```python
from build123d import *

# Parameters (mm, degrees)
SKETCH_1_W                   = 60
SKETCH_1_H                   = 20
EXTRUDE_1_DEPTH              = 20
SKETCH_2_W                   = 60
SKETCH_2_H                   = 40
EXTRUDE_2_DEPTH              = 5
SKETCH_3_W                   = 20
SKETCH_3_H                   = 5
EXTRUDE_3_DEPTH              = 20
HOLE_WIZARD_M4_2_D           = 4.5
HOLE_WIZARD_M4_2_CBORE_D     = 8
HOLE_WIZARD_M4_2_CBORE_DEPTH = 4
SKETCH_8_W                   = 15
SKETCH_8_H                   = 20
CUT_EXTRUDE_1_DEPTH          = 84.815273071
HOLE_WIZARD_M4_1_D           = 4.5
HOLE_WIZARD_M4_1_CBORE_D     = 8
HOLE_WIZARD_M4_1_CBORE_DEPTH = 4
SKETCH_10_W                  = 60
SKETCH_10_H                  = 5
EXTRUDE_4_DEPTH              = 80
SKETCH_11_W                  = 60
SKETCH_11_H                  = 5
EXTRUDE_5_DEPTH              = 20
FILLET_1_R                   = 20
SKETCH_12_W                  = 10
SKETCH_12_H                  = 5
CUT_EXTRUDE_2_DEPTH          = 129.937969582
SKETCH_13_W                  = 14
SKETCH_13_H                  = 20
CUT_EXTRUDE_3_DEPTH          = 35
SKETCH_14_W                  = 14
SKETCH_14_H                  = 3
EXTRUDE_6_DEPTH              = 20
HOLE_WIZARD_M4_1_2_D         = 4.6
HOLE_WIZARD_M4_1_2_DEPTH     = 5


with BuildPart() as part:
    # 스케치1 → 보스-돌출1 (new body)
    with BuildSketch(Plane.XY):
        Rectangle(SKETCH_1_W, SKETCH_1_H)
    extrude(amount=EXTRUDE_1_DEPTH)

    # 스케치2 → 보스-돌출2 (add)
    with BuildSketch(Plane.XZ.offset(10)):
        Rectangle(SKETCH_2_W, SKETCH_2_H)
    extrude(amount=EXTRUDE_2_DEPTH)

    # 스케치3 → 보스-돌출3 (add)
    with BuildSketch(Plane(origin=(30, 0, 0), x_dir=(0, 0, -1), z_dir=(1, 0, 0))):
        with Locations((10, -12.5)):
            Rectangle(SKETCH_3_W, SKETCH_3_H)
    extrude_3 = extrude(amount=EXTRUDE_3_DEPTH)

    # 대칭 복사1: 보스-돌출3 across plane
    add(extrude_3.mirror(Plane.ZY))

    # M4 소켓 머리 캡 나사용 카운터보어2 (through all)
    with Locations(Plane(origin=(0, -15, 0), x_dir=(-1, 0, 0), z_dir=(0, -1, 0))):
        with Locations((40, 10), (-40, 10)):
            CounterBoreHole(HOLE_WIZARD_M4_2_D / 2, HOLE_WIZARD_M4_2_CBORE_D / 2, HOLE_WIZARD_M4_2_CBORE_DEPTH)

    # 스케치8 → 컷-돌출1 (cut, through all)
    with BuildSketch(Plane(origin=(30, 0, 0), x_dir=(0, 0, -1), z_dir=(1, 0, 0))):
        with Locations((-12.5, 0)):
            Rectangle(SKETCH_8_W, SKETCH_8_H)
    extrude(amount=-CUT_EXTRUDE_1_DEPTH, mode=Mode.SUBTRACT)

    # Hole Wizard M4 _ _ _ _ _1 (through all)
    with Locations(Plane(origin=(0, -10, 0), x_dir=(1, 0, 0), z_dir=(0, 1, 0))):
        with Locations((-15, 10), (15, 10), (-15, -10), (15, -10)):
            CounterBoreHole(HOLE_WIZARD_M4_1_D / 2, HOLE_WIZARD_M4_1_CBORE_D / 2, HOLE_WIZARD_M4_1_CBORE_DEPTH)

    # 스케치10 → 보스-돌출4 (add)
    with BuildSketch(Plane.XY.offset(20)):
        with Locations((0, -12.5)):
            Rectangle(SKETCH_10_W, SKETCH_10_H)
    extrude(amount=EXTRUDE_4_DEPTH)

    # 스케치11 → 보스-돌출5 (add)
    with BuildSketch(Plane(origin=(0, -10, 0), x_dir=(1, 0, 0), z_dir=(0, 1, 0))):
        with Locations((0, -97.5)):
            Rectangle(SKETCH_11_W, SKETCH_11_H)
    extrude(amount=EXTRUDE_5_DEPTH)

    # 필렛1
    fillet_1_edges = [part.edges().sort_by_distance(p)[0] for p in [
        (0, -10, 95),
    ]]
    fillet(fillet_1_edges, radius=FILLET_1_R - 0.0001)  # a hair under: the kernel refuses the full size

    # 스케치12 → 컷-돌출2 (cut, through all)
    with BuildSketch(Plane.ZY.offset(30)):
        with Locations((95, -12.5)):
            Rectangle(SKETCH_12_W, SKETCH_12_H)
    extrude(amount=-CUT_EXTRUDE_2_DEPTH, mode=Mode.SUBTRACT)

    # 스케치13 → 컷-돌출3 (cut)
    with BuildSketch(Plane.XY.offset(60)):
        with Locations((-15, 0)):
            Rectangle(SKETCH_13_W, SKETCH_13_H)
        with Locations((15, 0)):
            Rectangle(SKETCH_13_W, SKETCH_13_H)
    extrude(amount=CUT_EXTRUDE_3_DEPTH, mode=Mode.SUBTRACT)

    # 스케치14 → 보스-돌출6 (add)
    with BuildSketch(Plane(origin=(0, 0, 95), x_dir=(-1, 0, 0), z_dir=(0, 0, -1))):
        with Locations((-15, -8.5)):
            Rectangle(SKETCH_14_W, SKETCH_14_H)
        with Locations((15, -8.5)):
            Rectangle(SKETCH_14_W, SKETCH_14_H)
    extrude(amount=EXTRUDE_6_DEPTH)

    # Hole Wizard M4 _ _1 2
    with Locations(Plane(origin=(0, 0, 95), x_dir=(-1, 0, 0), z_dir=(0, 0, -1))):
        with Locations((-15, 0), (15, 0)):
            Hole(HOLE_WIZARD_M4_1_2_D / 2, depth=HOLE_WIZARD_M4_1_2_DEPTH)


solid = part.part
```
Part model, mm, in its own coordinate system. A direction names the side the tool comes from. Round coordinates to 2 decimals unless told otherwise and drop trailing zeros. Loops run counter-clockwise (first coordinate to the right, second up) from the corner with the lowest first, then second, coordinate; pieces in that order, holes last. Notation, with made-up numbers: (30, 8.25) -> (47, 8.25) arc R13 ccw to (47, 20.25) -> close; hole circle Ø5 at (-16.75, 56). An arc over 180 degrees is marked (long way). Use one line per item in the form item = value. Start each with the question number.
Item 1: Band-saw the part on A-A (z = 10). List the corners of the cut face in (x, y), plus the area to 3 significant figures.
Item 2: Band-saw the part on B-B (x = -15). Give the number of separate pieces and of enclosed holes in the cut face, plus the area to 3 significant figures.
Item 3: Band-saw the part on D-D (y = -5.5). List the corners of the cut face in (x, z).
Item 4: Tool access for faces 4 (the flat face through (0, 0, 0)), 5 (the flat face through (-22, -8, 79)), 6 (the cylindrical face through (-36, -13, -10)): list every direction of +Z, -Z, +X, -X, +Y, -Y with a clear straight run to the whole face (end or side of a thin tool).
Item 5: Two-plate mould, pull along X, no slides. Class faces 1 (the flat face through (22, -8, 79)), 2 (the cylindrical face through (11, -12, -10)), 3 (the flat face through (0, -10, 40)): released by +X, released by -X, zero draft, split by the parting line, or undercut.
Item 6: Drill centre lines: line 1 along Z through (x, y) = (15, -12.85); line 2 along X through (y, z) = (-14.45, 10); line 3 along Y through (x, z) = (15, 97.05). Where is each one in solid material? Low to high.
Item 7: Drop flat-ended pins along their axis: pin 1 Ø4 at (x, y) = (-45, -12) entering from +Z; pin 2 Ø5 at (x, y) = (-0.5, 2.5) entering from -Z; pin 3 Ø8 at (x, z) = (3.5, 39) entering from +Y; pin 4 Ø10.5 at (x, z) = (-40, -10) entering from -Y. Give the stop position or say it passes through.
Item 8: Band-saw the part on C-C (x = 40). List the corners of the cut face in (y, z), plus the area to 3 significant figures.
Data:
q1.outline = (-30, -15) -> (-17.25, -15) -> (-17.25, -14) -> (-19, -14) -> (-19, -10) -> (-30, -10) -> close; (-12.75, -15) -> (12.75, -15) -> (12.75, -14) -> (11, -14) -> (11, -10) -> (-11, -10) -> (-11, -14) -> (-12.75, -14) -> close; (17.25, -15) -> (30, -15) -> (30, -10) -> (19, -10) -> (19, -14) -> (17.25, -14) -> close
q1.area = 227 mm^2
q2.separate_pieces = 4
q2.enclosed_holes = 0
q2.area = 714 mm^2
q3.outline = (-30, 0) -> (30, 0) -> (30, 5) -> (-30, 5) -> close; (-30, 87.64) -> (-22, 87.64) -> (-22, 95) -> (-8, 95) -> (-8, 87.64) -> (8, 87.64) -> (8, 95) -> (22, 95) -> (22, 87.64) -> (30, 87.64) -> (30, 100) -> (-30, 100) -> close
q4.face_4 = -Z, +X, -X, +Y
q4.face_5 = -X, +Y
q4.face_6 = -Y
q5.face_1 = released by +X
q5.face_2 = undercut
q5.face_3 = zero draft
q6.line_1 = -20 to -14, -6 to 6, 14 to 90
q6.line_2 = -30 to -17.25, -12.75 to 12.75, 17.25 to 30
q6.line_3 = -10 to -2.3, 2.3 to 10
q7.pin_1 = 0
q7.pin_2 = 0
q7.pin_3 = -10
q7.pin_4 = -15
q8.outline = (-15, -20) -> (-10, -20) -> (-10, -12.25) -> (-11, -12.25) -> (-11, -14) -> (-15, -14) -> close; (-15, -6) -> (-11, -6) -> (-11, -7.75) -> (-10, -7.75) -> (-10, 0) -> (-15, 0) -> close
q8.area = 63.5 mm^2
